Model file for the job. Use its own axes, mm. Coordinates: 2 decimals unless noted, no trailing zeros. Loops run counter-clockwise (first coordinate to the right, second up) from the corner with the lowest first, then second, coordinate; pieces in that order, holes last.
from build123d import *

# Parameters (mm, degrees)
SKETCH1_R                   = 3.9497
BOSS_EXTRUDE1_DEPTH         = 130.175
F_37_0_104_DIAMETER_HOLE1_D = 2.6416
CHAMFER1_SIZE               = 0.508


with BuildPart() as part:
    # Sketch1 → Boss-Extrude1 (new body)
    with BuildSketch(Plane.XY):
        Circle(SKETCH1_R)
    extrude(amount=BOSS_EXTRUDE1_DEPTH)

    # #37 (0.104) Diameter Hole1 (through all)
    with Locations(Plane(origin=(3.9497, 0, 0), x_dir=(0, 0, -1), z_dir=(1, 0, 0))):
        with Locations((-6.35, 0), (-123.825, 0)):
            Hole(F_37_0_104_DIAMETER_HOLE1_D / 2)

    # Chamfer1
    chamfer1_edges = [part.edges().sort_by_distance(p)[0] for p in [
        (-3.9497, 0, 0),
        (-3.9497, 0, 130.175),
    ]]
    chamfer(chamfer1_edges, length=CHAMFER1_SIZE)


solid = part.part
Q1. Mould opens along Z. For faces 1 (the cylindrical face through (-0.1, -0.8, 5.3)), 2 (the cylindrical face through (-0.856, -3.856, 64.183)), 3 (the flat face through (0, 0, 0)) say: +Z half, -Z half, draft (parallel to the pull), parting line (faces both ways), or undercut.
Answers:
face 1: undercut
face 2: draft
face 3: -Z half
Q2. Slice it at C-C (z = 16). List the corners of the cut face in (x, y), and give its area (3 significant figures).
Answers:
outline: circle Ø7.9 at (0, 0)
area: 49.0 mm2
Q3. Flat gauge pins, fed straight in: P1, Ø3.5, axis at y = 0, z = 6.35, coming from the -X side; P2, Ø1, axis at x = -3, z = 88.5, coming from the +Y side; P3, Ø1, axis at x = -2.5, z = 56, coming from the +Y side; P4, Ø2, axis at x = 1.5, z = 43.5, coming from the -Y side. Where does each tip first touch, or does it go through?
Answers:
P1: stops at x = -3.95
P2: stops at y = 3.06
P3: stops at y = 3.41
P4: stops at y = -3.92
Q4. Drill centre lines: line 1 (Z direction, x = 1, y = 0) (3 decimals); line 2 (Z direction, x = -0.5, y = -0.5) (1 decimal); line 3 (Y direction, x = 0.5, z = 6.35). Where is each one in solid material? Low to high.
Answers:
line 1: z = 0 to 5.029, 7.671 to 122.504, 125.146 to 130.175
line 2: z = 0 to 5.1, 7.6 to 122.6, 125 to 130.2
line 3: y = -3.92 to -1.32, 1.32 to 3.92
Q5. Slice it at A-A (y = 0). List the corners of the cut face in (x, z) (3 decimals), and give its area (3 significant figures).
Answers:
outline: (-3.95, 0.508) - (-3.442, 0) - (3.442, 0) - (3.95, 0.508) - (3.95, 5.029) - (-3.95, 5.029) - close; (-3.95, 7.671) - (3.95, 7.671) - (3.95, 122.504) - (-3.95, 122.504) - close; (-3.95, 125.146) - (3.95, 125.146) - (3.95, 129.667) - (3.442, 130.175) - (-3.442, 130.175) - (-3.95, 129.667) - close
area: 986 mm2
Q6. Slice it at B-B (x = 1.25). Count the separate pieces of the cut face and the enclosed holes in it, and give its area (3 significant figures).
Answers:
separate pieces: 1
enclosed holes: 2
area: 964 mm2
